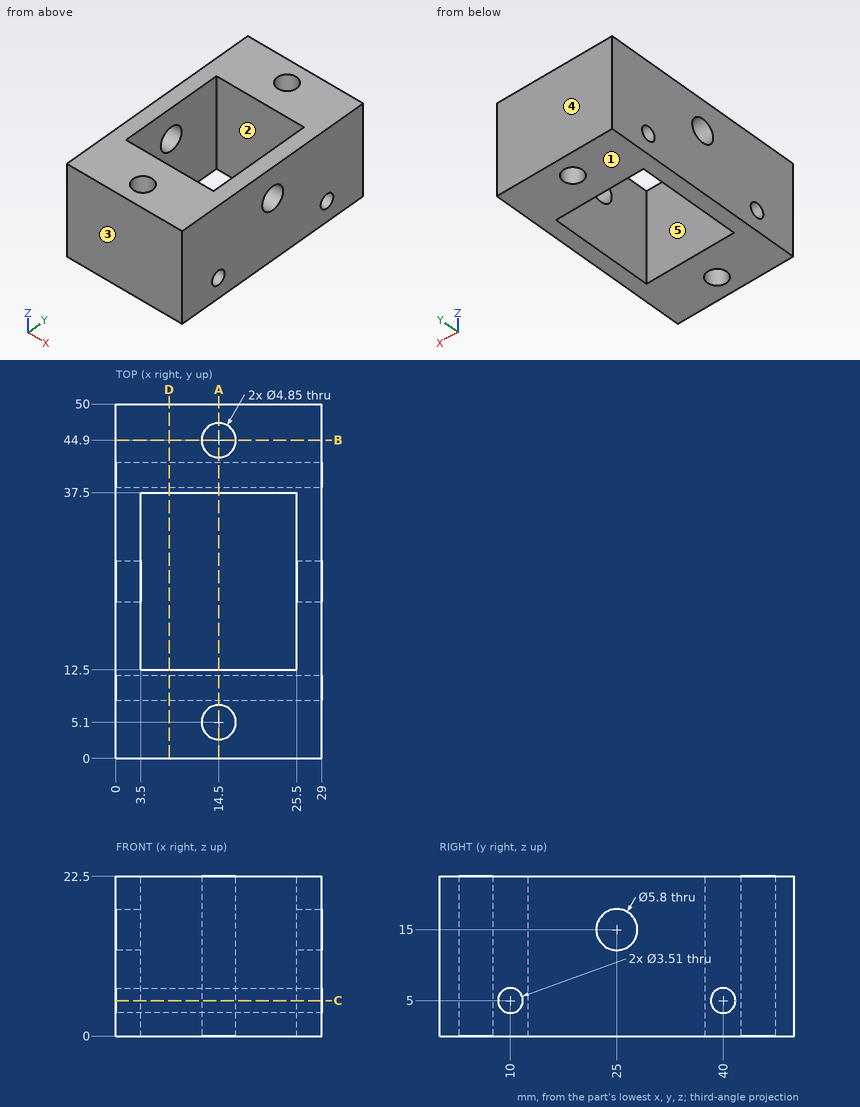
Geometry check sheet. Reference: drawing and pictorial views, mm from the part's lowest x, y, z. A direction names the side the tool comes from. Give positions to 0.01 mm unless a question says otherwise; leave off trailing zeros. Loops run counter-clockwise (first coordinate to the right, second up) from the corner with the lowest first, then second, coordinate; pieces in that order, holes last. Notation, with made-up numbers: (57, 85) - (89, 85) arc R36 ccw to (89, 120) - close; hole circle Ø4 at (-27, 50). An arc over 180 degrees is marked (long way). Use CSV: the item, a comma, the result in double quotes. Start each with the question number.
Q1. Section check D-D, the plane x = 7.5. Record the cut outline in (y, z) (3 decimals), and give its area (3 significant figures).
Q2. Section check C-C, the plane z = 5. Record the cut outline in (x, y) (3 decimals), and give its area (3 significant figures).
Q3. Release check for a two-part mould opening along Y. For the marked faces 3, 4 and 5 record: +Y half, -Y half, draft (parallel to the pull), parting line (faces both ways), or undercut.
Q4. Scan lines: probe 1 along Y at (x, z) = (12, 5) (3 decimals); probe 2 along Y at (x, z) = (14.5, 7) (3 decimals); probe 3 along Y at (x, z) = (1.8, 15). Record each from-to range of solid material in increasing order. Write a range as from..to.
Q5. Section check A-A, the plane x = 14.5. Record the cut outline in (y, z) (3 decimals).
Q6. Access from +Z, -Z, +X, -X, +Y, -Y to the whole of each face (thin tool, end or side, straight path). Record for the marked faces 1 and 2.
Q7. Section check B-B, the plane y = 44.9. Record the cut outline in (x, z) (3 decimals), and give its area (3 significant figures).
Findings below:
1,outline,"(0, 0) - (12.5, 0) - (12.5, 22.5) - (0, 22.5) - close; (37.5, 0) - (50, 0) - (50, 22.5) - (37.5, 22.5) - close; hole circle Ø3.51 at (10, 5); hole circle Ø3.51 at (40, 5)"
1,area,"543 mm^2"
2,outline,"(0, 0) - (29, 0) - (29, 8.245) - (0, 8.245) - close; (0, 11.755) - (29, 11.755) - (29, 38.245) - (0, 38.245) - close; (0, 41.755) - (29, 41.755) - (29, 50) - (0, 50) - close; hole (3.5, 12.5) - (25.5, 12.5) - (25.5, 37.5) - (3.5, 37.5) - close; hole circle Ø4.85 at (14.5, 5.1); hole circle Ø4.85 at (14.5, 44.9)"
2,area,"659 mm^2"
3,face 3,"-Y half"
3,face 4,"+Y half"
3,face 5,"undercut"
4,probe 1,"y = 0..8.245, 11.755..12.5, 37.5..38.245, 41.755..50"
4,probe 2,"y = 0..2.675, 7.525..12.5, 37.5..42.475, 47.325..50"
4,probe 3,"y = 0..22.1, 27.9..50"
5,outline,"(0, 0) - (2.675, 0) - (2.675, 22.5) - (0, 22.5) - close; (7.525, 0) - (12.5, 0) - (12.5, 22.5) - (7.525, 22.5) - close; (37.5, 0) - (42.475, 0) - (42.475, 22.5) - (37.5, 22.5) - close; (47.325, 0) - (50, 0) - (50, 22.5) - (47.325, 22.5) - close; hole circle Ø3.51 at (10, 5); hole circle Ø3.51 at (40, 5)"
6,face 1,"-Z, +X, -X, +Y, -Y"
6,face 2,"+Z, -Z"
7,outline,"(0, 0) - (12.075, 0) - (12.075, 22.5) - (0, 22.5) - close; (16.925, 0) - (29, 0) - (29, 22.5) - (16.925, 22.5) - close"
7,area,"543 mm^2"
